Part model, mm, in its own coordinate system. A direction names the side the tool comes from. Coordinates: 2 decimals unless noted, no trailing zeros. Order: outer loops, then holes, each group sorted by start corner. A loop starts at its lowest first (then second) coordinate and runs counter-clockwise, first axis right, second up. Notation, with made-up numbers: M -23,76 L -4,76 A21 cw -4,87 Z; hole C 75,-14.5 d9. An arc over 180 degrees is marked long. Answer in a Markdown table with one row per item. Add a question column.
Autodesk Inventor part; units mm, degrees
ref_plane "YZ Plane" through (0, 0, 0) normal (1, 0, 0) x (0, 1, 0)
ref_plane "XZ Plane" through (0, 0, 0) normal (0, 1, 0) x (-1, 0, 0)
ref_plane "XY Plane" through (0, 0, 0) normal (0, 0, 1) x (1, 0, 0)
sketch "Sketch1" plane through (0, 0, 0) normal (0, 1, 0) x (-1, 0, 0)
  line L0 (0, 0) -> (0, -153.89) construction
  line L1 (3, 0) -> (3, -153.89)
  line L2 (-3, -153.89) -> (-3, 0)
  arc A0 (3, 0) -> (-3, 0) centre (0, 0) ccw
  arc A1 (-3, -153.89) -> (3, -153.89) centre (0, -153.89) ccw
  circle A2 centre (0, 0) radius 1.1
  circle A3 centre (0, -153.89) radius 1.1
  circle A4 centre (0, -25.907) radius 1.1
  circle A5 centre (0, -127.773) radius 1.1
  arc A6 (3, -127.773) -> (3, -25.907) centre (-292.6448, -76.84) ccw
  arc A7 (-3, -127.773) -> (-3, -25.907) centre (-298.6448, -76.84) ccw
  point P0 (0, -76.945)
  dimension "d0" = 2.2
  dimension "d1" = 2.2
  dimension "d2" = 6
  dimension "d3" = 153.89
  dimension "d10" = 2.2
  dimension "d11" = 25.907
  dimension "d12" = 2.2
  dimension "d13" = 127.773
  dimension "d16" = 300
  dimension "d17" = 300
extrude "Extrusion1" add sketch "Sketch1" along normal blind 4 contours L1 A1 L2 A7 A0 | A6 L1
(1) Wall check: line 1 (X direction, y = 2.4, z = -153.89); line 2 (X direction, y = 1.6, z = -80.5); line 3 (X direction, y = 3, z = -8.5). Give the ranges that are in metal, low to high.
(2) Slice it at A-A (y = 0.8). List the corners of the cut face in (x, z).
(3) 3-axis set-ups, long thin cutter, end or side, ignore diameter. For faces 1 (the flat face through (-3, 2, -141)), 2 (the flat face through (3, 2, -13)), 3 (the flat face through (-3, 2, -13)): which of +Z, -Z, +X, -X, +Y, -Y reach the whole face in a straight line?
(4) Slice it at B-B (z = -23.5). List the corners of the cut face in (x, y).
(5) Drop flat-ended pins along their axis: P1, Ø2, axis at x = 0.5, z = -88, coming from the +Y side; P2, Ø1.5, axis at x = 0.5, z = -15, coming from the -Y side; P3, Ø2, axis at y = 3, z = -139.5, coming from the -X side. Give the stop position or say it passes through.
(6) Pull direction Z, two halves, no side cores. Call faces 4 (the flat face through (3, 2, -141)), 5 (the cylindrical face through (-0.07, 1.97, -156.89)), 6 (the cylindrical face through (-1.354, 1.972, -76.123)): pulls with the +Z half, pulls with the -Z half, needs draft (parallel to the pull), parting line crosses it, or undercut.
Computed:
| question | item | result |
|---|---|---|
| 1 | line 1 | x = -3 to -1.1, 1.1 to 3 |
| 1 | line 2 | x = -7.33 to -1.33 |
| 1 | line 3 | x = -3 to 3 |
| 2 | outline | M -3,-153.89 A3 ccw 3,-153.89 L 3,-127.77 A300 cw 3,-25.91 L 3,0 A3 ccw -3,0 L -3,-25.91 A300 ccw -3,-127.77 Z; hole C 0,-153.89 d2.2; hole C 0,-127.77 d2.2; hole C 0,-25.91 d2.2; hole C 0,0 d2.2 |
| 3 | face 1 | -Z, -X, +Y, -Y |
| 3 | face 2 | +Z, -Z, +X, +Y, -Y |
| 3 | face 3 | +Z, -X, +Y, -Y |
| 4 | outline | M -3,0 L 3,0 L 3,4 L -3,4 Z |
| 5 | P1 | passes through |
| 5 | P2 | stops at y = 0 |
| 5 | P3 | stops at x = -3 |
| 6 | face 4 | needs draft |
| 6 | face 5 | pulls with the -Z half |
| 6 | face 6 | undercut |
